Read the model definition and answer for the solid it produces. Units are mm, in the model's axes. Face numbers are marked on the shaded views. A direction names the side the tool comes from. Give positions to 0.01 mm unless a question says otherwise; leave off trailing zeros. Order: outer loops, then holes, each group sorted by start corner. A loop starts at its lowest first (then second) coordinate and runs counter-clockwise, first axis right, second up.
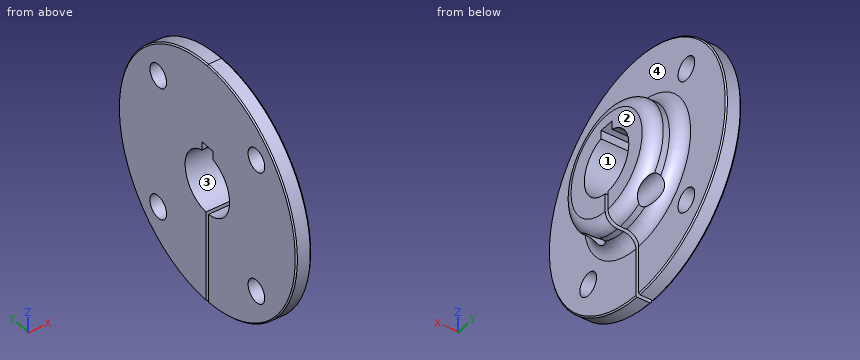
```python
from build123d import *

# Parameters (mm, degrees)
F2_R          = 5.08
F3_SIZE       = 0.508
F4_R          = 4.7625
F4_W          = 6.35
F4_H          = 6.35
F4_W_2        = 1.5875
F4_H_2        = 60.4483003783
F5_DEPTH      = 19.051
F6_R          = 3.96875
F7_DEPTH      = 50.801
F7_DEPTH_BACK = 50.801


with BuildPart() as f1:
    # F0 (on Front) → F1 (revolve)
    with BuildSketch(Plane.XZ):
        Polygon((0, 50.8), (0, 12.7), (19.05, 12.7), (19.05, 25.4), (6.35, 25.4), (6.35, 50.8), align=None)
    revolve(axis=Axis((9.525, 0, 0), (1, 0, 0)))

    # F2
    f2_edges = [f1.edges().sort_by_distance(p)[0] for p in [
        (19.05, 0, -25.4),
        (6.35, 0, -25.4),
    ]]
    fillet(f2_edges, radius=F2_R)

    # F3
    f3_edges = [f1.edges().sort_by_distance(p)[0] for p in [
        (6.35, 0, -50.8),
        (0, 0, -50.8),
    ]]
    chamfer(f3_edges, length=F3_SIZE)

    # F4 (on face) → F5 (cut, through all)
    with BuildSketch(Plane(origin=(0, 0, 0), x_dir=(0, -1, 0), z_dir=(-1, 0, 0))):
        with Locations((-28.0633003783, 28.0633003783)):
            Circle(F4_R)
        with Locations((-28.0633003783, -28.0633003783)):
            Circle(F4_R)
        with Locations((28.0633003783, -28.0633003783)):
            Circle(F4_R)
        with Locations((28.0633003783, 28.0633003783)):
            Circle(F4_R)
        with Locations((0, 12.7)):
            Rectangle(F4_W, F4_H)
        with Locations((0, -23.2391501892)):
            Rectangle(F4_W_2, F4_H_2)
    extrude(amount=-F5_DEPTH, mode=Mode.SUBTRACT)

    # F6 (on Front) → F7 (cut, two sides)
    with BuildSketch(Plane.XZ) as f7_sk:
        with Locations((12.7, -18.8722)):
            Circle(F6_R)
    extrude(amount=-F7_DEPTH, mode=Mode.SUBTRACT)
    extrude(f7_sk.sketch, amount=F7_DEPTH_BACK, mode=Mode.SUBTRACT)


solid = f1.part
```
1) The part is cut by section D-D on y = -5.5. Count the separate pieces of the cut face and the enclosed holes in it, and give its area (3 significant figures).
Final values:
separate pieces: 2
enclosed holes: 1
area: 785 mm2
2) A tool of negligible diameter and unlimited length cuts with its end or side. For the marked faces 1 and 2, from which of +Z, -Z, +X, -X, +Y, -Y can it reach the whole face along a straight path? Write none if from no direction.
Final values:
face 1: +X, -X
face 2: +Z, -Z, +X, +Y, -Y
3) The part is cut by section A-A on z = 0. Determine the outline of the cut face in (x, y), and give its area (3 significant figures).
Final values:
outline: (0, -50.29) - (0.51, -50.8) - (5.84, -50.8) - (6.35, -50.29) - (6.35, -30.48) arc R5.08 cw to (11.43, -25.4) - (13.97, -25.4) arc R5.08 ccw to (19.05, -20.32) - (19.05, -12.7) - (0, -12.7) - close; (0, 12.7) - (19.05, 12.7) - (19.05, 20.32) arc R5.08 ccw to (13.97, 25.4) - (11.43, 25.4) arc R5.08 cw to (6.35, 30.48) - (6.35, 50.29) - (5.84, 50.8) - (0.51, 50.8) - (0, 50.29) - close
area: 806 mm2
4) Given pin 1 (1.8 mm diameter, centred on x = 8.5, z = 14.5, fed in from +Y); pin 2 (1 mm diameter, centred on x = 6.5, y = 1.5, fed in from +Z); pin 3 (5 mm diameter, centred on y = -23.5, z = 39, fed in from +X); pin 4 (1 mm diameter, centred on y = 11.5, z = -1, fed in from -X), each flat-ended and moving along its own axis, determine where each tip first touches the part or whether it passes through.
Final values:
pin 1: stops at y = 23.07
pin 2: stops at z = 50.62
pin 3: stops at x = 6.35
pin 4: passes through
5) For a pull along Z with two mould halves and no side action, classify the marked faces 3 and 4 as released by +Z, released by -Z, zero draft, split by the parting line, or undercut.
Final values:
face 3: undercut
face 4: zero draft
6) The part is cut by section C-C on x = 4.5. Determine the outline of the cut face in (y, z) (1 decimal), and give its area (3 significant figures).
Final values:
outline: (-3.2, 12.3) - (-3.2, 15.9) - (3.2, 15.9) - (3.2, 12.3) arc R12.7 cw to (0.8, -12.7) - (0.8, -50.8) arc R50.8 ccw (long way) to (-0.8, -50.8) - (-0.8, -12.7) arc R12.7 cw to start; hole circle Ø9.5 at (-28.1, -28.1); hole circle Ø9.5 at (-28.1, 28.1); hole circle Ø9.5 at (28.1, -28.1); hole circle Ø9.5 at (28.1, 28.1)
area: 7,230 mm2
7) Consider L1, parallel to X at y = 45, z = 10; L2, parallel to Y at x = 14.75, z = -9; L3, parallel to Y at x = 7.75, z = -24. Determine where each line is inside the solid, lowest interval first.
Final values:
L1: x = 0 to 6.35
L2: y = -23.69 to -8.96, 8.96 to 23.69
L3: y = -12.32 to -0.79, 0.79 to 12.32
8) The part is cut by section B-B on x = 12.7. Determine the outline of the cut face in (y, z) (3 decimals).
Final values:
outline: (-20.568, -14.903) - (-0.794, -14.903) - (-0.794, -12.675) arc R12.7 cw to (-3.175, 12.297) - (-3.175, 15.875) - (3.175, 15.875) - (3.175, 12.297) arc R12.7 cw to (0.794, -12.675) - (0.794, -14.903) - (20.568, -14.903) arc R25.4 ccw (long way) to start; (-11.111, -22.841) arc R25.4 ccw to (-0.794, -25.388) - (-0.794, -22.841) - close; (0.794, -25.388) arc R25.4 ccw to (11.111, -22.841) - (0.794, -22.841) - close
